from build123d import *

# Parameters (mm, degrees)
SKETCH1_W                              = 142.9333456
SKETCH1_H                              = 72.120000116
SKETCH1_W_2                            = 126.000012266
SKETCH1_H_2                            = 64.500000116
BOSS_EXTRUDE1_DEPTH                    = 12.7
CUT_EXTRUDE1_DEPTH                     = 5.08
CUT_EXTRUDE2_DEPTH                     = 5.08
CUT_EXTRUDE3_DEPTH                     = 5.08
CHAMFER1_SIZE                          = 0.635
CUT_EXTRUDE4_DEPTH                     = 2.54
F_18_0_1695_DIAMETER_HOLE1_D           = 4.3053
F_18_0_1695_DIAMETER_HOLE1_DEPTH       = 3.81
F_18_0_1695_DIAMETER_HOLE1_CSINK_D     = 5.5753
F_18_0_1695_DIAMETER_HOLE1_CSINK_ANGLE = 90
BOSS_EXTRUDE2_DEPTH                    = 2.54
F_6_CLEARANCE_HOLE1_D                  = 4.3053
F_6_CLEARANCE_HOLE1_CSINK_D            = 6.6548
F_6_CLEARANCE_HOLE1_CSINK_ANGLE        = 90


with BuildPart() as part:
    # Sketch1 → Boss-Extrude1 (new body)
    with BuildSketch(Plane(origin=(0, 0, 0), x_dir=(0, 0, -1), z_dir=(1, 0, 0))):
        with Locations((0, -2.54)):
            Rectangle(SKETCH1_W, SKETCH1_H)
        Rectangle(SKETCH1_W_2, SKETCH1_H_2, mode=Mode.SUBTRACT)
    extrude(amount=-BOSS_EXTRUDE1_DEPTH)

    # Sketch2 → Cut-Extrude1 (cut)
    with BuildSketch(Plane(origin=(0, 33.520000058, 0), x_dir=(1, 0, 0), z_dir=(0, 1, 0))):
        Polygon((-3.175, 67.233339467), (-6.35, 64.058339467), (-9.525, 67.233339467), (-6.35, 70.408339467), align=None)
        Polygon((-3.175, -67.233339467), (-6.35, -70.408339467), (-9.525, -67.233339467), (-6.35, -64.058339467), align=None)
    extrude(amount=-CUT_EXTRUDE1_DEPTH, mode=Mode.SUBTRACT)

    # Sketch3 → Cut-Extrude2 (cut)
    with BuildSketch(Plane.ZY.offset(12.7)):
        Polygon((70.408339467, 25.053333392), (67.233339467, 21.878333392), (64.058339467, 25.053333392), (67.233339467, 28.228333392), align=None)
        Polygon((-64.058339467, -30.133333392), (-67.233339467, -33.308333392), (-70.408339467, -30.133333392), (-67.233339467, -26.958333392), align=None)
        Polygon((64.058339467, -30.133333392), (67.233339467, -26.958333392), (70.408339467, -30.133333392), (67.233339467, -33.308333392), align=None)
    extrude(amount=-CUT_EXTRUDE2_DEPTH, mode=Mode.SUBTRACT)

    # Sketch5 → Cut-Extrude3 (cut)
    with BuildSketch(Plane.XZ.offset(38.600000058)):
        Polygon((-4.233333333, -70.408339467), (-7.408333333, -67.233339467), (-4.233333333, -64.058339467), (-1.058333333, -67.233339467), align=None)
        Polygon((-4.233333333, 64.058339467), (-7.408333333, 67.233339467), (-4.233333333, 70.408339467), (-1.058333333, 67.233339467), align=None)
    extrude(amount=-CUT_EXTRUDE3_DEPTH, mode=Mode.SUBTRACT)

    # Chamfer1
    chamfer1_edges = [part.edges().sort_by_distance(p)[0] for p in [
        (-2.645833333, -33.520000058, -68.820839467),
        (-5.820833333, -33.520000058, -68.820839467),
        (-5.820833333, -33.520000058, -65.645839467),
        (-2.645833333, -33.520000058, -65.645839467),
        (-2.645833333, -38.600000058, -68.820839467),
        (-2.645833333, -38.600000058, -65.645839467),
        (-5.820833333, -38.600000058, -65.645839467),
        (-5.820833333, -38.600000058, -68.820839467),
        (-2.645833333, -33.520000058, 65.645839467),
        (-5.820833333, -33.520000058, 65.645839467),
        (-5.820833333, -33.520000058, 68.820839467),
        (-2.645833333, -33.520000058, 68.820839467),
        (-2.645833333, -38.600000058, 65.645839467),
        (-2.645833333, -38.600000058, 68.820839467),
        (-5.820833333, -38.600000058, 68.820839467),
        (-5.820833333, -38.600000058, 65.645839467),
        (-4.7625, 28.440000058, -68.820839467),
        (-4.7625, 28.440000058, -65.645839467),
        (-7.9375, 28.440000058, -65.645839467),
        (-7.9375, 28.440000058, -68.820839467),
        (-4.7625, 33.520000058, -68.820839467),
        (-7.9375, 33.520000058, -68.820839467),
        (-7.9375, 33.520000058, -65.645839467),
        (-4.7625, 33.520000058, -65.645839467),
        (-4.7625, 28.440000058, 65.645839467),
        (-4.7625, 28.440000058, 68.820839467),
        (-7.9375, 28.440000058, 68.820839467),
        (-7.9375, 28.440000058, 65.645839467),
        (-4.7625, 33.520000058, 65.645839467),
        (-7.9375, 33.520000058, 65.645839467),
        (-7.9375, 33.520000058, 68.820839467),
        (-4.7625, 33.520000058, 68.820839467),
        (-7.62, 26.640833392, 68.820839467),
        (-7.62, 23.465833392, 68.820839467),
        (-7.62, 23.465833392, 65.645839467),
        (-7.62, 26.640833392, 65.645839467),
        (-12.7, 26.640833392, 68.820839467),
        (-12.7, 26.640833392, 65.645839467),
        (-12.7, 23.465833392, 65.645839467),
        (-12.7, 23.465833392, 68.820839467),
        (-7.62, -28.545833392, -65.645839467),
        (-7.62, -31.720833392, -65.645839467),
        (-7.62, -31.720833392, -68.820839467),
        (-7.62, -28.545833392, -68.820839467),
        (-12.7, -28.545833392, -65.645839467),
        (-12.7, -28.545833392, -68.820839467),
        (-12.7, -31.720833392, -68.820839467),
        (-12.7, -31.720833392, -65.645839467),
        (-7.62, -31.720833392, 65.645839467),
        (-7.62, -28.545833392, 65.645839467),
        (-7.62, -28.545833392, 68.820839467),
        (-7.62, -31.720833392, 68.820839467),
        (-12.7, -31.720833392, 65.645839467),
        (-12.7, -31.720833392, 68.820839467),
        (-12.7, -28.545833392, 68.820839467),
        (-12.7, -28.545833392, 65.645839467),
    ]]
    chamfer(chamfer1_edges, length=CHAMFER1_SIZE)

    # Sketch6 → Cut-Extrude4 (cut)
    with BuildSketch(Plane(origin=(0, -32.250000058, 0), x_dir=(1, 0, 0), z_dir=(0, 1, 0))):
        with BuildLine():
            Line((-8.466666582, -55.126006133), (-12.7, -55.126006133))
            Line((-12.7, -55.126006133), (-12.7, -63.000006133))
            Line((-12.7, -63.000006133), (-8.466666582, -63.000006133))
            ThreePointArc((-8.466666582, -63.000006133), (-4.529666582, -59.063006133), (-8.466666582, -55.126006133))
        make_face()
    extrude(amount=-CUT_EXTRUDE4_DEPTH, mode=Mode.SUBTRACT)

    # #18 (0.1695) Diameter Hole1
    with Locations(Plane(origin=(0, -34.790000058, 0), x_dir=(1, 0, 0), z_dir=(0, 1, 0))):
        with Locations((-8.466666582, -59.063006133)):
            CounterSinkHole(F_18_0_1695_DIAMETER_HOLE1_D / 2, F_18_0_1695_DIAMETER_HOLE1_CSINK_D / 2, depth=F_18_0_1695_DIAMETER_HOLE1_DEPTH, counter_sink_angle=F_18_0_1695_DIAMETER_HOLE1_CSINK_ANGLE)

    # Sketch9 → Boss-Extrude2 (add)
    with BuildSketch(Plane(origin=(0, 0, 0), x_dir=(0, 0, -1), z_dir=(1, 0, 0))):
        Polygon((-63.000006133, 20.669993925), (-56.216595593, 20.669993925), (-51.42, 25.466589518), (-51.42, 32.250000058), (-63.000006133, 32.250000058), align=None)
        Polygon((-63.000006133, -20.669993925), (-56.216595593, -20.669993925), (-51.42, -25.466589518), (-51.42, -32.250000058), (-63.000006133, -32.250000058), align=None)
        Polygon((51.42, -32.250000058), (51.42, -25.466589518), (56.216595593, -20.669993925), (63.000006133, -20.669993925), (63.000006133, -32.250000058), align=None)
        Polygon((51.42, 32.250000058), (51.42, 25.466589518), (56.216595593, 20.669993925), (63.000006133, 20.669993925), (63.000006133, 32.250000058), align=None)
    extrude(amount=-BOSS_EXTRUDE2_DEPTH)

    # #6 Clearance Hole1 (through all)
    with Locations(Plane(origin=(0, 0, 0), x_dir=(0, 0, -1), z_dir=(1, 0, 0))):
        with Locations((-56.5, 25.75), (56.5, 25.75), (56.5, -25.75), (-56.5, -25.75)):
            CounterSinkHole(F_6_CLEARANCE_HOLE1_D / 2, F_6_CLEARANCE_HOLE1_CSINK_D / 2, counter_sink_angle=F_6_CLEARANCE_HOLE1_CSINK_ANGLE)


solid = part.part
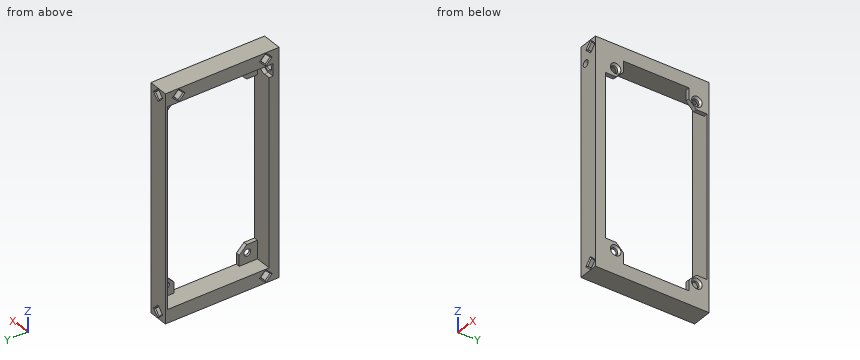
Design review of the part built by this model. Coordinates are the model's own, in mm. Round coordinates to 2 decimals unless told otherwise and drop trailing zeros. Loops run counter-clockwise (first coordinate to the right, second up) from the corner with the lowest first, then second, coordinate; pieces in that order, holes last. Notation, with made-up numbers: (-11.5, -23.5) - (47.5, -23.5) arc R31 cw to (47.5, 0.5) - close; hole circle Ø11 at (53.25, 68). An arc over 180 degrees is marked (long way). One line per question, with ' | ' between items.
1. Clearance check with flat-ended pins moving along their axes: P1, Ø3.5, axis at y = -25.75, z = -56.5, coming from the -X side; P2, Ø9.5, axis at y = -25.5, z = -56, coming from the -X side; P3, Ø1.4, axis at x = -5, z = -67.5, coming from the -Y side; P4, Ø1.4, axis at y = -29.5, z = -66, coming from the -X side. State where each tip first meets the part, or that it passes through.
Results are:
P1: passes through | P2: stops at x = -2.54 | P3: stops at y = -33.52 | P4: stops at x = -8.03
2. We need section A-A, the plane z = 17. State the section outline as (x, y) points, and give its area (3 significant figures).
Results are:
outline: (-12.7, -38.6) - (0, -38.6) - (0, -32.25) - (-12.7, -32.25) - close; (-12.7, 32.25) - (0, 32.25) - (0, 33.52) - (-12.7, 33.52) - close | area: 96.8 mm²
3. For L1, parallel to Z at x = -1.9, y = -25.75; L2, parallel to Y at x = -2.15, z = 56.5; L3, parallel to Z at x = -3, y = 13.5, list the stretches that pass through material, from the lowest coordinate up. Write a range as [from, to].
Results are:
L1: z = [-71.47, -58.65], [-54.35, -51.42], [51.42, 54.35], [58.65, 71.47] | L2: y = [-38.6, -27.9], [-23.6, -20.67], [20.67, 23.6], [27.9, 33.52] | L3: z = [-71.47, -63], [63, 71.47]
4. We need section B-B, the plane y = -2. State the section outline as (x, z) points, and give its area (3 significant figures).
Results are:
outline: (-12.7, -71.47) - (0, -71.47) - (0, -63) - (-12.7, -63) - close; (-12.7, 63) - (0, 63) - (0, 71.47) - (-12.7, 71.47) - close | area: 215 mm²
